```python
from build123d import *

# Parameters (mm, degrees)
F0_W     = 381
F0_H     = 254
F1_DEPTH = 254
F3_W     = 203.2
F3_H     = 101.6
F4_DEPTH = 25.4
F7_W     = 58.020108
F7_H     = 75.872456
F8_DEPTH = 254


with BuildPart() as f1:
    # F0 (on Top) → F1 (new body)
    with BuildSketch(Plane.XY):
        with Locations((-79.399429, -3.591057)):
            Rectangle(F0_W, F0_H)
        Polygon((263.500571, 0), (111.100571, 123.408943), (111.100571, -130.591057), align=None)
    extrude(amount=F1_DEPTH)

    # F3 (on face) → F4 (cut)
    with BuildSketch(Plane.XY.offset(254)):
        with Locations((-168.299429, 14.378742)):
            Rectangle(F3_W, F3_H)
    extrude(amount=-F4_DEPTH, mode=Mode.SUBTRACT)

    # F5 (on face) → F6 (revolve)
    with BuildSketch(Plane.XY.offset(254)):
        with BuildLine():
            Line((-269.899429, 276.197859), (-269.899429, 428.597859))
            ThreePointArc((-269.899429, 428.597859), (-346.099429, 352.397859), (-269.899429, 276.197859))
        make_face()
    revolve(axis=Axis((-3.199429, 0, 254), (-1, 0, 0)))

    # F7 (on face) → F8 (cut, through all)
    with BuildSketch(Plane.XY.offset(254)):
        with Locations((75.068335, 66.202429)):
            Rectangle(F7_W, F7_H)
        with Locations((-1.131665, 66.202429)):
            Rectangle(F7_W, F7_H)
        with Locations((-1.131665, -76.037571)):
            Rectangle(F7_W, F7_H)
        with Locations((75.068335, -76.037571)):
            Rectangle(F7_W, F7_H)
    extrude(amount=-F8_DEPTH, mode=Mode.SUBTRACT)


solid = f1.part
```
Verification items for the finished model (mm, model axes). A direction names the side the tool comes from. Round coordinates to 2 decimals unless told otherwise and drop trailing zeros. Write each loop counter-clockwise with the first axis right and the second up, starting at its lowest first coordinate (ties: lowest second). Pieces come first, ordered by that corner, then holes. Notation, with made-up numbers: (-31, 28.5) - (-27, 28.5) arc R14 cw to (-27, 54.5) - close; hole circle Ø6 at (67, -21.75). An arc over 180 degrees is marked (long way). Answer as a JSON object with one key per item and string values. Group by question number.
Q1. Tool access check on faces 4 (the flat face through (186.234, -66.21, 125.222)), 5 (the flat face through (-66, -2, 0)), 6 (the flat face through (188.37, 60.84, 125.22)), 7 (the flat face through (75, 28.266, 129)), 8 (the flat face through (-170, -36.421, 241)). Record the directions out of +Z, -Z, +X, -X, +Y, -Y that give a thin tool (end or side, any length) a straight path to the whole face; none if there is none.
Q2. Mould release check, pull along X, two halves, no side actions. Record for faces 1 (the flat face through (-82, -130.591, 125)), 2 (the flat face through (-269.899, -5, 125)), 3 (the flat face through (75, -38.101, 129)): released by +X, released by -X, zero draft, split by the parting line, or undercut.
Q3. Section check D-D, the plane x = 144.5. Enter the section's corners in (y, z).
Q4. Section check B-B, the plane x = -239. Enter the section's corners in (y, z), plus the area to 3 significant figures.
Q5. Section check A-A, the plane x = 69.5. Enter the section's corners in (y, z).
Q6. Section check C-C, the plane z = 38. Give the number of separate pieces and of enclosed holes in the cut face, plus the area to 3 significant figures.
Q7. Go/stop test with flat-tipped pins: pin 1 Ø23 at (y, z) = (71.5, 79) entering from -X; pin 2 Ø5 at (y, z) = (273.5, 538) entering from -X; pin 3 Ø6 at (x, z) = (-89, 33.5) entering from -Y. Record where each tip stops, or that it passes through.
Q8. Thickness scan on line 1 (Y direction, x = -155, z = 88); line 2 (Z direction, x = 130, y = 9); line 3 (Y direction, x = -295.5, z = 168). Record the ranges inside material, lowest first.
Found:
{
 "1": {"face 4": "+Z, -Z, +X, -Y", "face 5": "-Z, +X, +Y, -Y", "face 6": "+Z, -Z, +X, +Y", "face 7": "+Z, -Z", "face 8": "+Z, -X"},
 "2": {"face 1": "zero draft", "face 2": "released by -X", "face 3": "undercut"},
 "3": {"outline": "(-101.97, 0) - (96.36, 0) - (96.36, 254) - (-101.97, 254) - close"},
 "4": {"outline": "(-130.59, 0) - (123.41, 0) - (123.41, 254) - (65.18, 254) - (65.18, 228.6) - (-36.42, 228.6) - (-36.42, 254) - (-130.59, 254) - close", "area": "61,900 mm^2"},
 "5": {"outline": "(-130.59, 0) - (-113.97, 0) - (-113.97, 254) - (-130.59, 254) - close; (-38.1, 0) - (28.27, 0) - (28.27, 254) - (-38.1, 254) - close; (104.14, 0) - (123.41, 0) - (123.41, 254) - (104.14, 254) - close"},
 "6": {"separate pieces": "3", "enclosed holes": "4", "area": "122,000 mm^2"},
 "7": {"pin 1": "stops at x = -269.9", "pin 2": "stops at x = -335.13", "pin 3": "stops at y = -130.59"},
 "8": {"line 1": "y = -130.59 to 123.41", "line 2": "z = 0 to 254", "line 3": "y = -415.36 to -267.12, 267.12 to 415.36"}
}
